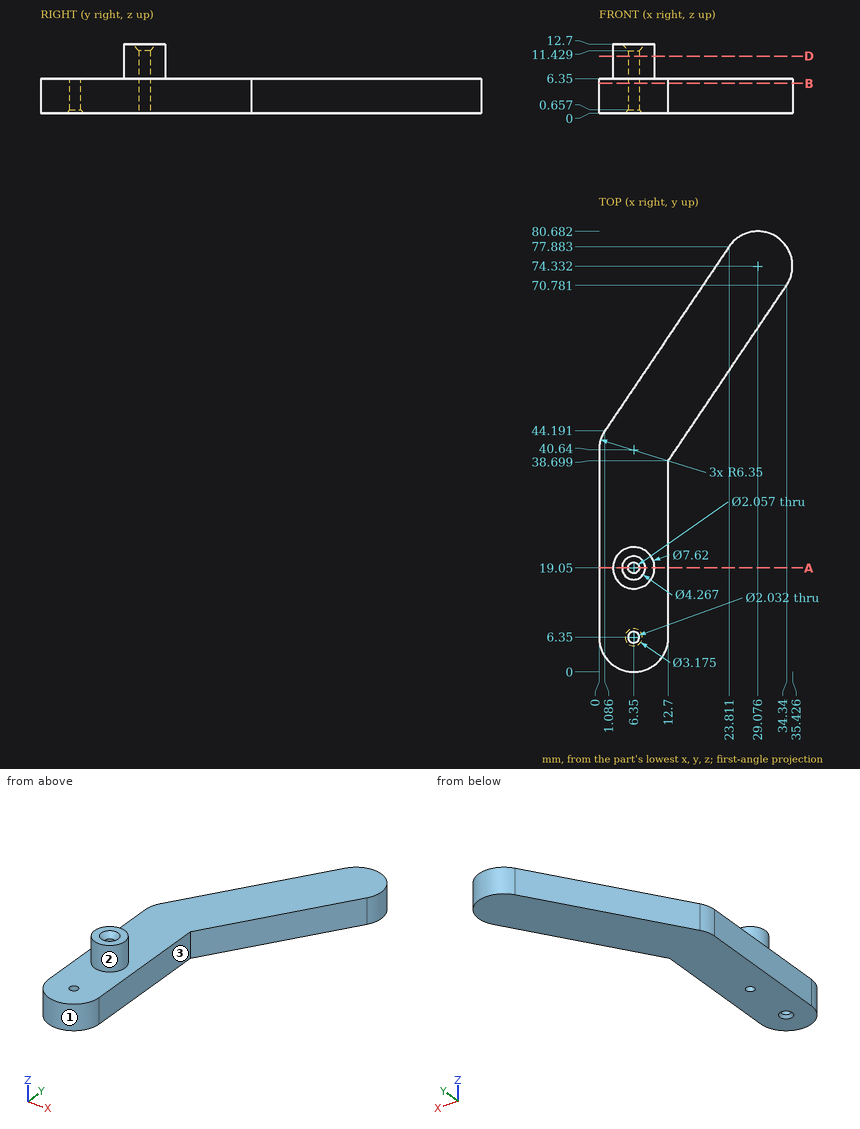
Design review of the part shown in the three views and the two pictorial views. Dimensions are in mm from the part's minimum x, y and z. A direction names the side the tool comes from. Round coordinates to 2 decimals unless told otherwise and drop trailing zeros. Loops run counter-clockwise (first coordinate to the right, second up) from the corner with the lowest first, then second, coordinate; pieces in that order, holes last.
(1) We need section B-B (z = 5.5). State how many separate pieces and enclosed holes the cut face has, plus the area to 3 significant figures.
Returned:
separate pieces: 1
enclosed holes: 2
area: 1,070 mm2
(2) We need section D-D (z = 10.5). Give the boundary of the cut face in (x, y), plus the area to 3 significant figures.
Returned:
outline: circle Ø7.62 at (6.35, 19.05); hole circle Ø2.06 at (6.35, 19.05)
area: 42.3 mm2
(3) Tool access review of the marked faces 1, 2 and 3: name each direction out of +Z, -Z, +X, -X, +Y, -Y from which nothing blocks a thin tool from reaching the whole face with its end or side.
Returned:
face 1: +Z, -Z, -Y
face 2: +Z
face 3: +Z, -Z, +X, -Y
(4) Clearance check with flat-ended pins moving along their axes: P1, Ø2.5, axis at x = 6.35, y = 6.35, coming from the -Z side; P2, Ø17.5, axis at x = 20, y = 46.5, coming from the +Z side; P3, Ø2, axis at x = 21.5, z = 6.5, coming from the +Y side. State where each tip first meets the part, or that it passes through.
Returned:
P1: stops at z = 0.39
P2: stops at z = 6.35
P3: stops at y = 75.92
(5) Wall thickness on line 1 along Y through (x, z) = (6.35, 8); line 2 along X through (y, z) = (19.05, 3.5); line 3 along Y through (x, z) = (6.35, 4.5) (1 decimal): over which ranges is each line inside the solid? List them lowest first.
Returned:
line 1: y = 15.24 to 18.02, 20.08 to 22.86
line 2: x = 0 to 5.32, 7.38 to 12.7
line 3: y = 0 to 5.3, 7.4 to 18, 20.1 to 52
(6) We need section A-A (y = 19.05). Give the boundary of the cut face in (x, z).
Returned:
outline: (0, 0) - (5.32, 0) - (5.32, 11.43) - (4.22, 12.7) - (2.54, 12.7) - (2.54, 6.35) - (0, 6.35) - close; (7.38, 0) - (12.7, 0) - (12.7, 6.35) - (10.16, 6.35) - (10.16, 12.7) - (8.48, 12.7) - (7.38, 11.43) - close
